Autodesk Inventor part; units mm, degrees
ref_plane "YZ Plane" through (0, 0, 0) normal (1, 0, 0) x (0, 1, 0)
ref_plane "XZ Plane" through (0, 0, 0) normal (0, 1, 0) x (-1, 0, 0)
ref_plane "XY Plane" through (0, 0, 0) normal (0, 0, 1) x (1, 0, 0)
sketch "Skizze1" plane through (0, 0, 0) normal (0, 1, 0) x (-1, 0, 0)
  line L0 (0, 0) -> (0, -445)
  line L1 (20, -465) -> (130, -465)
  line L2 (150, -485) -> (150, -645)
  line L3 (130, -665) -> (-130, -665)
  line L4 (-150, -685) -> (-150, -845)
  line L5 (-130, -865) -> (0, -865)
  line L6 (0, -865) -> (0, -1330)
  arc A0 (150, -485) -> (130, -465) centre (130, -485) ccw
  arc A1 (130, -665) -> (150, -645) centre (130, -645) ccw
  arc A2 (0, -445) -> (20, -465) centre (20, -445) ccw
  arc A3 (-130, -665) -> (-150, -685) centre (-130, -685) ccw
  arc A4 (-150, -845) -> (-130, -865) centre (-130, -845) ccw
  point P0 (0, -465)
  point P1 (150, -465)
  point P2 (150, -665)
  point P3 (-150, -665)
  point P4 (-150, -865)
  dimension "lange1" = 465
  dimension "d1" = 150
  dimension "d2" = 200
  dimension "d3" = 300
  dimension "d4" = 200
  dimension "lange2" = 465
  dimension "d6" = 20
sketch "Skizze2" plane through (0, 0, 0) normal (0, 0, 1) x (1, 0, 0)
  circle A0 centre (0, 0) radius 10
  dimension "durchmesser" = 20
sweep "Sweeping1" add profiles "Skizze2" path "Skizze1"
properties part number "Trittstange" material "Edelstahl"
Work out the finished part from the listing and answer in its coordinate system (mm). Give positions to 0.01 mm unless a question says otherwise; leave off trailing zeros. Write each loop counter-clockwise with the first axis right and the second up, starting at its lowest first coordinate (ties: lowest second). Pieces come first, ordered by that corner, then holes. Notation, with made-up numbers: (67.25, -36.75) -> (94.25, -36.75) arc R27 cw to (94.25, -0.75) -> close; hole circle Ø3 at (57.25, 52.25). An arc over 180 degrees is marked (long way). Write item = value, one per line.
Q1. Section C-C on z = -832 is taken. Determine the outline of the cut face in (x, y).
Computed values:
outline = circle Ø20 at (150, 0)
Q2. Section A-A on x = -94.5 is taken. Determine the outline of the cut face in (y, z), and give its area (3 significant figures).
Computed values:
outline = circle Ø20 at (0, -665); circle Ø20 at (0, -465)
area = 628 mm^2
Q3. Flat-ended cylindrical pins translate along their axes: pin 1 Ø5 at (x, y) = (102, 0.5) entering from -Z; pin 2 Ø1.5 at (y, z) = (-1.5, -212) entering from +X; pin 3 Ø1 at (x, y) = (73, 1.5) entering from +Z. Find the tip coordinate at first contact, or state that the pin passes through.
Computed values:
pin_1 = -875
pin_2 = 9.97
pin_3 = -655.05
Q4. Section B-B on y = 5.75 is taken. Determine the outline of the cut face in (x, z).
Computed values:
outline = (-158.18, -645) arc R28.18 ccw to (-130, -673.18) -> (130, -673.18) arc R11.82 cw to (141.82, -685) -> (141.82, -845) arc R11.82 cw to (130, -856.82) -> (-8.18, -856.82) -> (-8.18, -1330) -> (8.18, -1330) -> (8.18, -873.18) -> (130, -873.18) arc R28.18 ccw to (158.18, -845) -> (158.18, -685) arc R28.18 ccw to (130, -656.82) -> (-130, -656.82) arc R11.82 cw to (-141.82, -645) -> (-141.82, -485) arc R11.82 cw to (-130, -473.18) -> (-20, -473.18) arc R28.18 ccw to (8.18, -445) -> (8.18, 0) -> (-8.18, 0) -> (-8.18, -445) arc R11.82 cw to (-20, -456.82) -> (-130, -456.82) arc R28.18 ccw to (-158.18, -485) -> close
Q5. Consider line 1 along Z through (x, y) = (-96, -1.5); line 2 along Z through (x, y) = (-2, 6); line 3 along Z through (x, y) = (-34, -0.25). Determine where each line is inside the solid, lowest interval first.
Computed values:
line_1 = -674.89 to -655.11, -474.89 to -455.11
line_2 = -1330 to -857, -673 to -657, -466.45 to 0
line_3 = -675 to -655, -475 to -455
